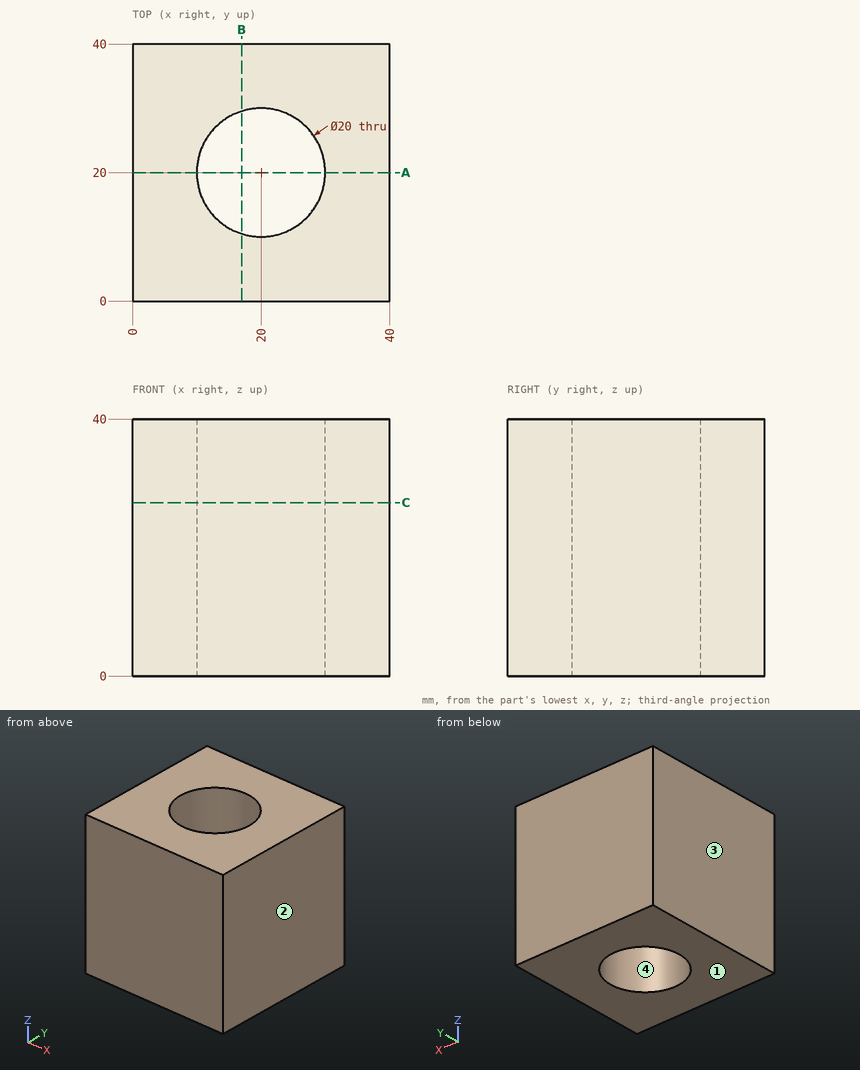
Can you work these out from the drawing? Everything is in mm from the part's minimum corner. Coordinates: 2 decimals unless noted, no trailing zeros. Loops run counter-clockwise (first coordinate to the right, second up) from the corner with the lowest first, then second, coordinate; pieces in that order, holes last.
1) Imagine slicing it at C-C (z = 27). List the corners of the cut face in (x, y) for me.
Reported:
outline: (0, 0) - (40, 0) - (40, 40) - (0, 40) - close; hole circle Ø20 at (20, 20)
2) Thinking about a two-plate mould opening in X: for the marked faces 1, 2, 3 and 4, which applies, released by +X, released by -X, zero draft, split by the parting line, or undercut?
Reported:
face 1: zero draft
face 2: released by +X
face 3: released by -X
face 4: undercut
3) Imagine slicing it at A-A (y = 20). List the corners of the cut face in (x, z) for me.
Reported:
outline: (0, 0) - (10, 0) - (10, 40) - (0, 40) - close; (30, 0) - (40, 0) - (40, 40) - (30, 40) - close
4) Imagine slicing it at B-B (x = 17). List the corners of the cut face in (y, z) for me, and give its area (3 significant figures).
Reported:
outline: (0, 0) - (10.46, 0) - (10.46, 40) - (0, 40) - close; (29.54, 0) - (40, 0) - (40, 40) - (29.54, 40) - close
area: 837 mm2
5) Will these pins go through, and if not, where does the flat tip stop? pin 1 Ø4 at (y, z) = (12.5, 13.5) entering from -X; pin 2 Ø16 at (x, y) = (20, 20) entering from -Z.
Reported:
pin 1: stops at x = 0
pin 2: passes through
6) Please list where these lines run through material, in increasing order: line 1 along Y through (x, z) = (20.5, 36); line 2 along X through (y, z) = (17, 28.5); line 3 along X through (y, z) = (14, 21.5).
Reported:
line 1: y = 0 to 10.01, 29.99 to 40
line 2: x = 0 to 10.46, 29.54 to 40
line 3: x = 0 to 12, 28 to 40
